For this review, take the finished solid that the model builds, in its own axes (mm). A direction names the side the tool comes from. Round coordinates to 2 decimals unless told otherwise and drop trailing zeros. Write each loop counter-clockwise with the first axis right and the second up, starting at its lowest first coordinate (ties: lowest second). Pieces come first, ordered by that corner, then holes. Notation, with made-up numbers: (51, -15.5) -> (96, -15.5) arc R32 cw to (96, 16.5) -> close; hole circle Ø10 at (73.5, 43). An arc over 180 degrees is marked (long way). Answer as CSV lines item,"result". Start each with the question number.
Item 1: For pin 1 Ø1 at (y, z) = (-10.5, 1) entering from -X; pin 2 Ø0.9 at (x, z) = (-22, 1) entering from +Y; pin 3 Ø1 at (x, z) = (-18.5, 1) entering from -Y, all flat-tipped, find the tip position at first contact; note any pin that passes through.
Item 2: Take a section at C-C on x = 0. Give the boundary of the cut face in (y, z), then the cut area to 4 significant figures.
Item 3: Mouldability with a two-part tool opening along Y and no side actions: class faces 1 (the cylindrical face through (-1.5, 0.07, 1.48)), 2 (the cylindrical face through (12.6, -79.14, 1.52)), 3 (the flat face through (13.5, -34, 1)), 4 (the flat face through (-21, -37.5, 1)) as +Y half, -Y half, draft (parallel to the pull), parting line (faces both ways), or undercut.
Item 4: Machinability: for faces 5 (the flat face through (-22.5, 0, 1)), 6 (the flat face through (-12.5, -72, 1)), 7 (the cylindrical face through (-21.64, -11.6, 1.52)), 8 (the flat face through (-22.5, -50, 1)), which of the approach directions +Z, -Z, +X, -X, +Y, -Y give a long, thin tool a straight path to every point of the face, cutting with its end or side? Answer none if there is none.
Item 5: Take a section at B-B on z = 0.9. Give the boundary of the cut face in (x, y).
Item 6: Take a section at D-D on y = -20. Give the boundary of the cut face in (x, z).
Item 7: Take a section at A-A on y = 0. Give the boundary of the cut face in (x, z), then the cut area to 3 significant figures.
Item 8: Wall thickness on probe 1 along Y at (x, z) = (0, 0.9); probe 2 along Y at (x, z) = (-17.5, 1.15); probe 3 along X at (y, z) = (-54, 1.9): over which ranges is each line inside the solid? List them lowest first. Write a range as from..to.
```python
from build123d import *

# Parameters (mm, degrees)
SKETCH_1_R      = 1.5
SKETCH_1_W      = 15
SKETCH_1_H      = 15
EXTRUDE_1_DEPTH = 3
FILLET_1_R      = 5
FILLET_2_R      = 3


with BuildPart() as part:
    # 草图1 → 凸台-拉伸1 (new body)
    with BuildSketch(Plane.XY):
        Polygon((13.5, -80), (13.5, 12.5), (-22.5, 12.5), (-22.5, -12.5), (-12.5, -12.5), (-12.5, -37.5), (-27.5, -37.5), (-27.5, -62.5), (-12.5, -62.5), (-12.5, -80), align=None)
        Circle(SKETCH_1_R, mode=Mode.SUBTRACT)
        with Locations((0, -20)):
            Circle(SKETCH_1_R, mode=Mode.SUBTRACT)
        with Locations((0, -68)):
            Circle(SKETCH_1_R, mode=Mode.SUBTRACT)
        with Locations((-17.5, 0)):
            Circle(SKETCH_1_R, mode=Mode.SUBTRACT)
        with Locations((-15, -50)):
            Rectangle(SKETCH_1_W, SKETCH_1_H, mode=Mode.SUBTRACT)
    extrude(amount=EXTRUDE_1_DEPTH)

    # 圆角1
    fillet_1_edges = [part.edges().sort_by_distance(p)[0] for p in [
        (-12.5, -62.5, 1.5),
        (-12.5, -37.5, 1.5),
        (-12.5, -12.5, 1.5),
    ]]
    fillet(fillet_1_edges, radius=FILLET_1_R)

    # 圆角2
    fillet_2_edges = [part.edges().sort_by_distance(p)[0] for p in [
        (13.5, 12.5, 1.5),
        (13.5, -80, 1.5),
        (-12.5, -80, 1.5),
        (-27.5, -62.5, 1.5),
        (-27.5, -37.5, 1.5),
        (-22.5, -12.5, 1.5),
        (-22.5, 12.5, 1.5),
    ]]
    fillet(fillet_2_edges, radius=FILLET_2_R)


solid = part.part
```
Output values:
1,pin 1,"stops at x = -22.46"
1,pin 2,"stops at y = 11.69"
1,pin 3,"stops at y = -62.5"
2,outline,"(-80, 0) -> (-69.5, 0) -> (-69.5, 3) -> (-80, 3) -> close; (-66.5, 0) -> (-21.5, 0) -> (-21.5, 3) -> (-66.5, 3) -> close; (-18.5, 0) -> (-1.5, 0) -> (-1.5, 3) -> (-18.5, 3) -> close; (1.5, 0) -> (12.5, 0) -> (12.5, 3) -> (1.5, 3) -> close"
2,area,"250.5 mm^2"
3,face 1,"undercut"
3,face 2,"-Y half"
3,face 3,"draft"
3,face 4,"undercut"
4,face 5,"+Z, -Z, -X, +Y"
4,face 6,"+Z, -Z, -X, -Y"
4,face 7,"+Z, -Z, -X"
4,face 8,"+Z, -Z"
5,outline,"(-27.5, -59.5) arc R3 ccw to (-24.5, -62.5) -> (-17.5, -62.5) arc R5 cw to (-12.5, -67.5) -> (-12.5, -77) arc R3 ccw to (-9.5, -80) -> (10.5, -80) arc R3 ccw to (13.5, -77) -> (13.5, 9.5) arc R3 ccw to (10.5, 12.5) -> (-19.5, 12.5) arc R3 ccw to (-22.5, 9.5) -> (-22.5, -9.5) arc R3 ccw to (-19.5, -12.5) -> (-17.5, -12.5) arc R5 cw to (-12.5, -17.5) -> (-12.5, -32.5) arc R5 cw to (-17.5, -37.5) -> (-24.5, -37.5) arc R3 ccw to (-27.5, -40.5) -> close; hole (-22.5, -57.5) -> (-7.5, -57.5) -> (-7.5, -42.5) -> (-22.5, -42.5) -> close; hole circle Ø3 at (-17.5, 0); hole circle Ø3 at (0, -68); hole circle Ø3 at (0, -20); hole circle Ø3 at (0, 0)"
6,outline,"(-12.5, 0) -> (-1.5, 0) -> (-1.5, 3) -> (-12.5, 3) -> close; (1.5, 0) -> (13.5, 0) -> (13.5, 3) -> (1.5, 3) -> close"
7,outline,"(-22.5, 0) -> (-19, 0) -> (-19, 3) -> (-22.5, 3) -> close; (-16, 0) -> (-1.5, 0) -> (-1.5, 3) -> (-16, 3) -> close; (1.5, 0) -> (13.5, 0) -> (13.5, 3) -> (1.5, 3) -> close"
7,area,"90.0 mm^2"
8,probe 1,"y = -80..-69.5, -66.5..-21.5, -18.5..-1.5, 1.5..12.5"
8,probe 2,"y = -62.5..-57.5, -42.5..-37.5, -12.5..-1.5, 1.5..12.5"
8,probe 3,"x = -27.5..-22.5, -7.5..13.5"
